Part model, mm, in its own coordinate system. A direction names the side the tool comes from. Give positions to 0.01 mm unless a question says otherwise; leave off trailing zeros. Order: outer loops, then holes, each group sorted by start corner. A loop starts at its lowest first (then second) coordinate and runs counter-clockwise, first axis right, second up. Notation, with made-up numbers: (22.25, 8) - (48.25, 8) arc R8 cw to (48.25, 16) - close; hole circle Ø1 at (-31.5, -23). An arc over 180 degrees is marked (long way). One line per item, written item: value.
```python
from build123d import *

# Parameters (mm, degrees)
SKETCH1_R           = 3
BOSS_EXTRUDE1_DEPTH = 100


with BuildPart() as part:
    # Sketch1 → Boss-Extrude1 (new body)
    with BuildSketch(Plane(origin=(0, 0, 0), x_dir=(1, 0, 0), z_dir=(0, 1, 0))):
        Circle(SKETCH1_R)
    extrude(amount=BOSS_EXTRUDE1_DEPTH)

    # Sketch3 → M3x0.5 Tapped Hole1 (revolve, cut)
    with BuildSketch(Plane(origin=(0, 0, 0), x_dir=(0, 0, -1), z_dir=(1, 0, 0))):
        Polygon((0, 0), (0, 5.751075774), (1.25, 5), (1.25, 0.275), (1.525, 0), align=None)
    m3x0_5_tapped_hole1 = revolve(axis=Axis((0, -6.35, 0), (0, 1, 0)), mode=Mode.SUBTRACT)

    # Mirror1: M3x0.5 Tapped Hole1 across plane
    add(m3x0_5_tapped_hole1.mirror(Plane.ZX.offset(50)), mode=Mode.SUBTRACT)


solid = part.part
```
1) Cut at A-A, the plane y = 36.5. Give the cut face in (x, z).
Outcome:
outline: circle Ø6 at (0, 0)
2) Pin check, flat tips, straight feed: pin 1 (2 mm diameter, centred on x = 0, z = 0, fed in from +Y); pin 2 (2 mm diameter, centred on y = 85.5, z = -2, fed in from -X); pin 3 (1.5 mm diameter, centred on y = 22.5, z = 1, fed in from +X). Stop position of each tip, or through.
Outcome:
pin 1: stops at y = 94.85
pin 2: stops at x = -2.83
pin 3: stops at x = 2.99
3) Which spindle directions (+Z, -Z, +X, -X, +Y, -Y) get a long thin tool onto all of the face, cutting with end or side? Do faces 1 (the flat face through (1.3, 0, 1.3)), 2 (the cylindrical face through (1.22, 97.4, 0.27)), 3 (the cylindrical face through (1.22, 2.6, 0.27)). Say none if no direction does.
Outcome:
face 1: +Z, -Z, +X, -X, -Y
face 2: +Y
face 3: -Y
4) Drill centre lines: line 1 along Z through (x, y) = (0, 96.7); line 2 along Z through (x, y) = (-0.3, 89.5). Where is each one in solid material? Low to high. Write a range as from..to.
Outcome:
line 1: z = -3..-1.25, 1.25..3
line 2: z = -2.98..2.98
5) Mould opens along X. For faces 4 (the cylindrical face through (-3, 49, 0)), 5 (the conical face through (0.21, 5.62, 0.05)), 6 (the flat face through (1.3, 100, 1.3)) say: released by +X, released by -X, zero draft, split by the parting line, or undercut.
Outcome:
face 4: split by the parting line
face 5: undercut
face 6: zero draft
